Could you check a few things on this model? Use its own coordinates, in mm. Round coordinates to 2 decimals unless told otherwise and drop trailing zeros. Write each loop counter-clockwise with the first axis right and the second up, starting at its lowest first coordinate (ties: lowest second). Pieces come first, ordered by that corner, then holes. Notation, with made-up numbers: (37, -26) -> (57, -26) arc R24 cw to (57, 1) -> close; hole circle Ø6 at (-28, -21.5). An arc over 180 degrees is marked (long way). Return JSON: item names as keys, results as strings.
from build123d import *

# Parameters (mm, degrees)
BOSS_EXTRUDE1_DEPTH  = 3.175
FILLET1_R            = 1.5875
SKETCH2_W            = 85.216
SKETCH2_H            = 12.7
BOSS_EXTRUDE2_DEPTH  = 3.175
FILLET2_R            = 1.5875
M4_CLEARANCE_HOLE1_D = 4.5
CUT_EXTRUDE1_START   = -3.175
SKETCH5_W            = 9.525
SKETCH5_H            = 1.5875
SKETCH5_W_2          = 10.541
SKETCH5_H_2          = 2.6035
CUT_EXTRUDE1_DEPTH   = 3.175


with BuildPart() as part:
    # Sketch1 → Boss-Extrude1 (new body)
    with BuildSketch(Plane(origin=(0, 0, 0), x_dir=(1, 0, 0), z_dir=(0, 1, 0))):
        with BuildLine():
            Line((-101.6, 0), (-101.6, -5.08))
            Line((-101.6, -5.08), (-1.894344313, -12.557924177))
            ThreePointArc((-1.894344313, -12.557924177), (-11.442635346, -5.50963668), (-10.998522628, 6.35))
            Line((-10.998522628, 6.35), (-101.6, 6.35))
            Line((-101.6, 6.35), (-101.6, 0))
        make_face()
    extrude(amount=BOSS_EXTRUDE1_DEPTH)

    # Fillet1
    fillet1_edges = [part.edges().sort_by_distance(p)[0] for p in [
        (-10.998522628, 1.5875, -6.35),
        (-1.894344313, 1.5875, 12.557924177),
    ]]
    fillet(fillet1_edges, radius=FILLET1_R)

    # Sketch2 → Boss-Extrude2 (add)
    with BuildSketch(Plane(origin=(0, 3.175, 0), x_dir=(1, 0, 0), z_dir=(0, 1, 0))):
        with Locations((-58.992, 12.7)):
            Rectangle(SKETCH2_W, SKETCH2_H)
    extrude(amount=-BOSS_EXTRUDE2_DEPTH)

    # Fillet2
    fillet2_edges = [part.edges().sort_by_distance(p)[0] for p in [
        (-101.6, 1.5875, -19.05),
        (-16.384, 1.5875, -19.05),
        (-16.384, 1.5875, -6.35),
        (-101.6, 1.5875, 5.08),
    ]]
    fillet(fillet2_edges, radius=FILLET2_R)

    # M4 Clearance Hole1 (through all)
    with Locations(Plane(origin=(0, 3.175, 0), x_dir=(1, 0, 0), z_dir=(0, 1, 0))):
        with Locations((-80.296, 12.7), (-58.992, 12.7), (-37.688, 12.7)):
            Hole(M4_CLEARANCE_HOLE1_D / 2)

    # Sketch5 → Cut-Extrude1 (cut)
    with BuildSketch(Plane(origin=(0, 3.175, 0), x_dir=(1, 0, 0), z_dir=(0, 1, 0)).offset(CUT_EXTRUDE1_START)):
        with Locations((-96.8375, -0.79375)):
            Rectangle(SKETCH5_W, SKETCH5_H)
        Polygon((-101.6, 0), (-92.075, 0), (-92.075, -1.5875), (-101.6, -1.5875), (-101.6, -2.0955), (-91.567, -2.0955), (-91.567, 0.508), (-101.6, 0.508), align=None)
        with Locations((-57.15, -0.79375)):
            Rectangle(SKETCH5_W_2, SKETCH5_H_2)
        with BuildLine():
            Line((-22.733, -2.0955), (-12.525928299, -2.0955))
            ThreePointArc((-12.525928299, -2.0955), (-12.674906095, -0.797969605), (-12.689835933, 0.508))
            Line((-12.689835933, 0.508), (-22.733, 0.508))
            Line((-22.733, 0.508), (-22.733, -2.0955))
        make_face()
    extrude(amount=CUT_EXTRUDE1_DEPTH, mode=Mode.SUBTRACT)


solid = part.part
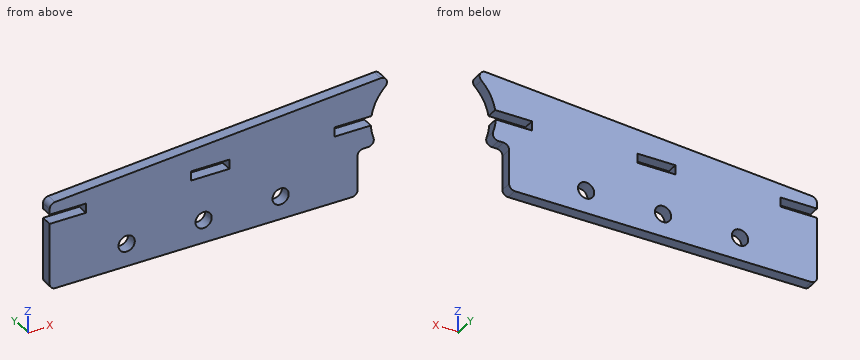
1) I want a section at D-D, the plane z = -5.5. Please give me the cut outline in (x, y) (3 decimals), and give its area (3 significant figures).
Return value:
{"outline": "(-101.6, 0) -> (-12.065, 0) -> (-12.065, 3.175) -> (-101.6, 3.175) -> close", "area": "284 mm²"}
2) Will these pins go through, and if not, where does the flat tip stop? pin 1 Ø1 at (x, y) = (-30.5, 0.5) entering from +Z; pin 2 Ø3 at (x, z) = (-82, -12) entering from -Y; pin 3 Ø0.8 at (y, z) = (1.5, 1) entering from -X; pin 4 Ø2.5 at (x, z) = (-58.992, -12.7) entering from +Y.
Return value:
{"pin 1": "z = 10.45", "pin 2": "y = 0", "pin 3": "x = -91.57", "pin 4": "through"}
3) I want a section at B-B, the plane y = 2.2. Count the separate pieces of the cut face and the enclosed holes in it, and give its area (3 significant figures).
Return value:
{"separate pieces": "1", "enclosed holes": "4", "area": "2,290 mm²"}
4) I want a section at C-C, the plane x = -90. Please give me the cut outline in (y, z) (3 decimals), and give its area (3 significant figures).
Return value:
{"outline": "(0, -19.05) -> (3.175, -19.05) -> (3.175, 5.95) -> (0, 5.95) -> close", "area": "79.4 mm²"}
5) I want a section at A-A, the plane z = -12.7. Please give me the cut outline in (x, y) (3 decimals).
Return value:
{"outline": "(-101.6, 0) -> (-82.546, 0) -> (-82.546, 3.175) -> (-101.6, 3.175) -> close; (-78.046, 0) -> (-61.242, 0) -> (-61.242, 3.175) -> (-78.046, 3.175) -> close; (-56.742, 0) -> (-39.938, 0) -> (-39.938, 3.175) -> (-56.742, 3.175) -> close; (-35.438, 0) -> (-16.384, 0) -> (-16.384, 3.175) -> (-35.438, 3.175) -> close"}
6) If I drill on probe 1 along X at (y, z) = (2.3, -12.7); probe 2 along X at (y, z) = (1.7, -10); probe 3 along X at (y, z) = (0.5, -11.5), over which ranges is the centre line in solid material (lowest first)? Write a range as [from, to].
Return value:
{"probe 1": "[-101.6, -82.55], [-78.05, -61.24], [-56.74, -39.94], [-35.44, -16.38]", "probe 2": "[-101.6, -16.38]", "probe 3": "[-101.6, -82.2], [-78.39, -60.9], [-57.09, -39.59], [-35.78, -16.38]"}
